Read the model definition and answer for the solid it produces. Units are mm, in the model's axes. Round coordinates to 2 decimals unless told otherwise and drop trailing zeros. Order: outer loops, then holes, each group sorted by start corner. A loop starts at its lowest first (then second) coordinate and runs counter-clockwise, first axis right, second up.
from build123d import *

# Parameters (mm, degrees)
F0_W     = 16.115269
F0_H     = 4.244756
F2_DEPTH = 29.323
F1_R     = 0.981148
F3_DEPTH = 42.4
F4_R     = 4.015374
F5_DEPTH = 25


with BuildPart() as f2:
    # F0 (on Front) → F2 (new body)
    with BuildSketch(Plane.XZ):
        with Locations((8.057634, 2.122378)):
            Rectangle(F0_W, F0_H)
    extrude(amount=-F2_DEPTH)

    # F1 (on face) → F3 (cut)
    with BuildSketch(Plane.XZ):
        with Locations((14.192748, 2.187148)):
            Circle(F1_R)
        with BuildLine():
            ThreePointArc((8.330639, 2.130213), (9.369746, 1.175413), (10.353437, 2.187214))
            ThreePointArc((10.353437, 2.187214), (9.312723, 3.199015), (8.330639, 2.130213))
        make_face()
    extrude(amount=-F3_DEPTH, mode=Mode.SUBTRACT)

    # F4 (on face) → F5 (cut)
    with BuildSketch(Plane.XY.offset(4.244756)):
        with Locations((7.023575, 14.6615)):
            Circle(F4_R)
    extrude(amount=-F5_DEPTH, mode=Mode.SUBTRACT)


solid = f2.part
Q1. A cutting plane is placed at B-B, the plane x = 9.5. Give the vertices of the cut face in (y, z), plus the area to 3 significant figures.
Outcome:
outline: (0, 0) - (11.5, 0) - (11.5, 1.19) - (0, 1.19) - close; (0, 3.19) - (11.5, 3.19) - (11.5, 4.24) - (0, 4.24) - close; (17.82, 0) - (29.32, 0) - (29.32, 1.19) - (17.82, 1.19) - close; (17.82, 3.19) - (29.32, 3.19) - (29.32, 4.24) - (17.82, 4.24) - close
area: 51.6 mm2
Q2. Straight lines are drawn through the part: probe 1 along X at (y, z) = (28, 2.15); probe 2 along X at (y, z) = (12.75, 2.5); probe 3 along Z at (x, y) = (14.25, 4). For each, find the intervals that lie inside material, in ascending order.
Outcome:
probe 1: x = 0 to 8.33, 10.35 to 13.21, 15.17 to 16.12
probe 2: x = 0 to 3.49, 10.55 to 13.26, 15.12 to 16.12
probe 3: z = 0 to 1.21, 3.17 to 4.24
Q3. A cutting plane is placed at A-A, the plane y = 17.25. Give the vertices of the cut face in (x, z).
Outcome:
outline: (0, 0) - (3.95, 0) - (3.95, 4.24) - (0, 4.24) - close; (10.09, 0) - (16.12, 0) - (16.12, 4.24) - (10.09, 4.24) - (10.09, 2.86) arc R1.01 cw to (10.35, 2.19) arc R1.01 cw to (10.09, 1.51) - close; hole circle Ø1.96 at (14.19, 2.19)
Q4. A cutting plane is placed at C-C, the plane z = 2.55. Give the vertices of the cut face in (x, y), plus the area to 3 significant figures.
Outcome:
outline: (0, 0) - (8.4, 0) - (8.4, 10.89) arc R4.02 cw (long way) to (8.4, 18.43) - (8.4, 29.32) - (0, 29.32) - close; (10.29, 0) - (13.28, 0) - (13.28, 29.32) - (10.29, 29.32) - (10.29, 17) arc R4.02 cw to (10.29, 12.32) - close; (15.1, 0) - (16.12, 0) - (16.12, 29.32) - (15.1, 29.32) - close
area: 325 mm2
Q5. A flat-ended cylindrical pin translates along its axis: pin 1 (5 mm diameter, centred on x = 7.02, y = 14.66, fed in from +Z). Find the tip coordinate at first contact, or state that the pin passes through.
Outcome:
pin 1: passes through
Q6. A cutting plane is placed at D-D, the plane x = 7.25. Give the vertices of the cut face in (y, z).
Outcome:
outline: (0, 0) - (10.65, 0) - (10.65, 4.24) - (0, 4.24) - close; (18.67, 0) - (29.32, 0) - (29.32, 4.24) - (18.67, 4.24) - close
Q7. For a pull along Y with two mould halves and no side action, classify faces 1 (the face through (0, 14, 2)), 2 (the face through (8, 0, 2)), 3 (the face through (8, 29.323, 2)), 4 (the face through (3.837, 12.218, 2.152)) as released by +Y, released by -Y, zero draft, split by the parting line, or undercut.
Outcome:
face 1: zero draft
face 2: released by -Y
face 3: released by +Y
face 4: undercut
